```python
from build123d import *

# Parameters (mm, degrees)
SKETCH1_W           = 23.75
SKETCH1_H           = 27.75
BOSS_EXTRUDE1_DEPTH = 5
SKETCH2_R           = 3.95
BOSS_EXTRUDE2_DEPTH = 20
FILLET1_R           = 3.45
FILLET2_R           = 2
CHAMFER1_SIZE       = 5


with BuildPart() as part:
    # Sketch1 → Boss-Extrude1 (new body)
    with BuildSketch(Plane(origin=(0, 0, 0), x_dir=(1, 0, 0), z_dir=(0, 1, 0))):
        Rectangle(SKETCH1_W, SKETCH1_H)
    extrude(amount=BOSS_EXTRUDE1_DEPTH)

    # Sketch2 → Boss-Extrude2 (add)
    with BuildSketch(Plane(origin=(0, 5, 0), x_dir=(1, 0, 0), z_dir=(0, 1, 0))):
        with Locations(Location((0, 8, 0), (0, 0, 90))):
            Circle(SKETCH2_R)
    extrude(amount=BOSS_EXTRUDE2_DEPTH)

    # Fillet1
    fillet1_edges = [part.edges().sort_by_distance(p)[0] for p in [
        (0, 25, -4.05),
    ]]
    fillet(fillet1_edges, radius=FILLET1_R)

    # Fillet2
    fillet2_edges = [part.edges().sort_by_distance(p)[0] for p in [
        (0, 5, -4.05),
    ]]
    fillet(fillet2_edges, radius=FILLET2_R)

    # Chamfer1
    chamfer1_edges = [part.edges().sort_by_distance(p)[0] for p in [
        (-11.875, 2.5, -13.875),
        (11.875, 2.5, -13.875),
    ]]
    chamfer(chamfer1_edges, length=CHAMFER1_SIZE)


solid = part.part
```
Geometry: final body of the model. Coordinates: model frame, mm. A direction names the side the tool comes from. Give positions to 0.01 mm unless a question says otherwise; leave off trailing zeros. Write each loop counter-clockwise with the first axis right and the second up, starting at its lowest first coordinate (ties: lowest second). Pieces come first, ordered by that corner, then holes.
1. Pin query (flat end, axial travel): P1, Ø7, axis at x = 2.5, z = 3, coming from the +Y side; P2, Ø5, axis at x = -3, y = 9, coming from the -Z side. Return the tip coordinate at first contact, or that it passes through.
2. Reachability of faces 1 (the cylindrical face through (-0.174, 14.172, -4.054)), 2 (the flat face through (0, 2, -13.875)) from +Z, -Z, +X, -X, +Y, -Y: full face, straight path, thin tool, end or side. Return the list, or none.
3. Section query B-B, the plane z = 2.75. Return loops of the section in (x, y) (3 decimals), then the cut area to 3 significant figures.
4. Section query A-A, the plane y = 2.75. Return loops of the section in (x, z) (3 decimals), then the cut area to 3 significant figures.
5. Section query C-C, the plane x = -10. Return loops of the section in (y, z) (3 decimals), then the cut area to 3 significant figures.
6. Line query: probe 1 along Y at (x, z) = (-9, 12.25); probe 2 along Z at (x, y) = (-3.5, 21); probe 3 along Z at (x, y) = (-1.5, 16). Output: solid intervals per line, ascending.
Computed:
1. P1: stops at y = 5
1. P2: stops at z = -11.92
2. face 1: +Y
2. face 2: -Z, +X, -X, +Y, -Y
3. outline: (-11.875, 0) - (11.875, 0) - (11.875, 5) - (-11.875, 5) - close
3. area: 119 mm2
4. outline: (-11.875, -8.875) - (-6.875, -13.875) - (6.875, -13.875) - (11.875, -8.875) - (11.875, 13.875) - (-11.875, 13.875) - close
4. area: 634 mm2
5. outline: (0, -10.75) - (5, -10.75) - (5, 13.875) - (0, 13.875) - close
5. area: 123 mm2
6. probe 1: y = 0 to 5
6. probe 2: z = -9.83 to -6.17
6. probe 3: z = -11.65 to -4.35
